For this review, take the finished solid that the model builds, in its own axes (mm). A direction names the side the tool comes from. Round coordinates to 2 decimals unless told otherwise and drop trailing zeros. Order: outer loops, then holes, each group sorted by start corner. A loop starts at its lowest first (then second) coordinate and runs counter-clockwise, first axis right, second up. Notation, with made-up numbers: M 75.25,50 L 110.25,50 A17 ccw 110.25,79 Z; hole C 38,-20 d1. An arc over 180 degrees is marked long. Answer in a Markdown table with one row per item. Add a question column.
Autodesk Inventor part; units mm, degrees
ref_plane "YZ Plane" through (0, 0, 0) normal (1, 0, 0) x (0, 1, 0)
ref_plane "XZ Plane" through (0, 0, 0) normal (0, 1, 0) x (-1, 0, 0)
ref_plane "XY Plane" through (0, 0, 0) normal (0, 0, 1) x (1, 0, 0)
sketch "スケッチ1" plane through (0, 0, 0) normal (0, 0, 1) x (1, 0, 0)
  circle A0 centre (0, 0) radius 25
  dimension "d0" = 50
extrude "押し出し1" add sketch "スケッチ1" along normal blind 3
sketch "スケッチ2" plane through (0, 0, 3) normal (0, 0, 1) x (1, 0, 0)
  circle A0 centre (0, 0) radius 20
  dimension "d3" = 40
extrude "押し出し2" add sketch "スケッチ2" along normal blind 40
sketch "スケッチ3" plane through (0, 0, 43) normal (0, 0, 1) x (1, 0, 0)
  circle A0 centre (0, 0) radius 25
  dimension "d6" = 50
extrude "押し出し3" add sketch "スケッチ3" along normal blind 3
sketch "スケッチ4" plane through (0, 0, 46) normal (0, 0, 1) x (1, 0, 0)
  circle A0 centre (0, 0) radius 2.5
  dimension "d9" = 5
hole "穴1" at (0, 0, 46) direction (0, 0, -1) diameter 5 depth 46
equation "\"BendRadius\" = Thickness"
equation "\"BendReliefWidth\" = Thickness"
equation "\"BendReliefDepth\" = 0.5 * Thickness"
equation "\"CornerReliefSize\" = 4 * Thickness"
equation "\"MinimumRemnant\" = 2 * Thickness"
equation "\"TransitionRadius\" = BendRadius"
equation "\"JacobiRadiusSize\" = BendRadius"
equation "\"GapSize\" = Thickness"
properties part number "nhk10"
1. Consider section A-A on y = 0. Write out the cut boundary in (x, z).
2. Consider section D-D on y = -18.5. Write out the cut boundary in (x, z), plus the area to 3 significant figures.
3. For faces 1 (the cylindrical face through (23.846, -7.509, 1.479)), 2 (the flat face through (-11, 17, 3)), list the 3-axis set-ups (+Z, -Z, +X, -X, +Y, -Y) from which the entire face can be reached by the end or side of a thin tool; tool diameter is ignored.
4. Consider section C-C on z = 39. Write out the cut boundary in (x, y), plus the area to 3 significant figures.
5. To check wall thickness, follow probe 1 along Y at (x, z) = (0, 29); probe 2 along Z at (x, y) = (19.5, 8); probe 3 along Y at (x, z) = (4.5, 30). State the ranges of each line that lie inside material, in increasing order. Write a range as [from, to].
6. The part is to be moulded in two halves that separate along Z. For faces 3 (the cylindrical face through (2.44, 0.54, 22.68)), 4 (the flat face through (0, -5, 0)), 5 (the cylindrical face through (-4.336, 19.524, 22.72)), say which applies: pulls with the +Z half, pulls with the -Z half, needs draft (parallel to the pull), parting line crosses it, or undercut.
7. Clearance check with flat-ended pins moving along their axes: pin 1 Ø12 at (y, z) = (14.5, 34.5) entering from +X; pin 2 Ø5 at (y, z) = (1, 39) entering from +X; pin 3 Ø12 at (y, z) = (-19, 26.5) entering from +X. State where each tip first meets the part, or that it passes through.
Solved:
| question | item | result |
|---|---|---|
| 1 | outline | M -25,0 L -2.5,0 L -2.5,46 L -25,46 L -25,43 L -20,43 L -20,3 L -25,3 Z; M 2.5,0 L 25,0 L 25,3 L 20,3 L 20,43 L 25,43 L 25,46 L 2.5,46 Z |
| 2 | outline | M -16.82,0 L 16.82,0 L 16.82,3 L 7.6,3 L 7.6,43 L 16.82,43 L 16.82,46 L -16.82,46 L -16.82,43 L -7.6,43 L -7.6,3 L -16.82,3 Z |
| 2 | area | 810 mm^2 |
| 3 | face 1 | +Z, -Z |
| 3 | face 2 | none |
| 4 | outline | C 0,0 d40; hole C 0,0 d5 |
| 4 | area | 1,240 mm^2 |
| 5 | probe 1 | y = [-20, -2.5], [2.5, 20] |
| 5 | probe 2 | z = [0, 3], [43, 46] |
| 5 | probe 3 | y = [-19.49, 19.49] |
| 6 | face 3 | needs draft |
| 6 | face 4 | pulls with the -Z half |
| 6 | face 5 | undercut |
| 7 | pin 1 | stops at x = 18.1 |
| 7 | pin 2 | stops at x = 20 |
| 7 | pin 3 | stops at x = 15.2 |
